Here's how the part is built. I have some questions about the finished solid (model axes, mm). Face numbers are marked on the shaded views. A direction names the side the tool comes from. Coordinates: 2 decimals unless noted, no trailing zeros. Order: outer loops, then holes, each group sorted by start corner. A loop starts at its lowest first (then second) coordinate and runs counter-clockwise, first axis right, second up. Notation, with made-up numbers: (-3, 2) - (4, 2) arc R34 ccw to (4, 33) - close; hole circle Ø5 at (-8, -10.5). An arc over 180 degrees is marked (long way). Answer in a Markdown table with one row per item. Add a question column.
Item 1: If I drill on line 1 along Z through (x, y) = (32, 17) (3 decimals); line 2 along Y through (x, z) = (2, -38.1) (3 decimals); line 3 along X through (y, z) = (35.5, 15.5) (3 decimals), over which ranges is the centre line in solid material (lowest first)? Write a range as from..to.
Item 2: I want a section at D-D (z = 38.1). Please give me the cut outline in (x, y) (3 decimals), plus the area to 3 significant figures.
Item 3: I want a section at A-A (z = -40). Please give me the cut outline in (x, y) (3 decimals).
Item 4: Thinking about a two-plate mould opening in Z: for the marked faces 1, 2 and 3, which applies, +Z half, -Z half, draft (parallel to the pull), parting line (faces both ways), or undercut?
Item 5: Will these pins go through, and if not, where does the flat tip stop? pin 1 Ø5 at (y, z) = (34.5, -36) entering from -X; pin 2 Ø8 at (x, z) = (22.5, 41.5) entering from +Y (3 decimals); pin 3 Ø12.5 at (y, z) = (53, 4) entering from +X (3 decimals).
Item 6: I want a section at B-B (x = 11). Please give me the cut outline in (y, z) (3 decimals).
Item 7: On a 3-axis mill with a long thin cutter (end or side, diameter ignored), from which of +Z, -Z, +X, -X, +Y, -Y can I reach the whole of each face in a straight line? I mean the marked faces 4, 5 and 6. Say none if no direction works.
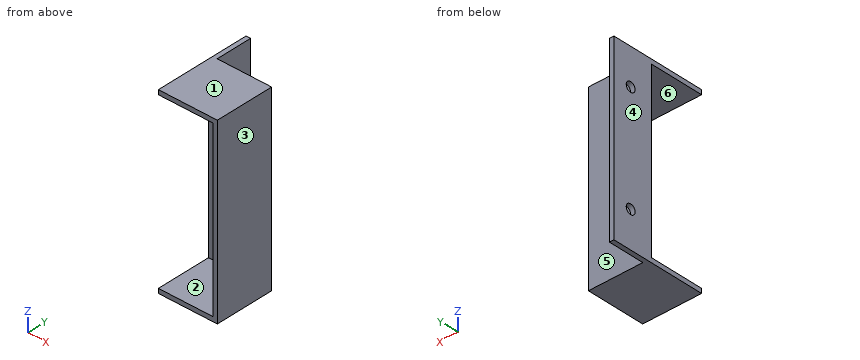
Autodesk Inventor part; units mm, degrees
ref_plane "YZ Plane" through (0, 0, 0) normal (1, 0, 0) x (0, 1, 0)
ref_plane "XZ Plane" through (0, 0, 0) normal (0, 1, 0) x (-1, 0, 0)
ref_plane "XY Plane" through (0, 0, 0) normal (0, 0, 1) x (1, 0, 0)
sketch "Sketch1" plane through (0, 0, 0) normal (0, 0, 1) x (1, 0, 0)
  line L0 (0, 66.675) -> (0, 38.1)
  line L1 (0, 66.675) -> (3.175, 66.675)
  line L2 (3.175, 66.675) -> (3.175, 41.275)
  line L3 (3.175, 41.275) -> (41.275, 41.275)
  line L4 (41.275, 41.275) -> (41.275, 0)
  line L5 (41.275, 0) -> (38.1, 0)
  line L6 (38.1, 0) -> (38.1, 38.1)
  line L7 (38.1, 38.1) -> (0, 38.1)
  point P0 (0, 0)
  dimension "d0" = 3.175
  dimension "d1" = 3.175
  dimension "d2" = 3.175
  dimension "d3" = 38.1
  dimension "d4" = 38.1
  dimension "d5" = 25.4
extrude "Extrusion1" add sketch "Sketch1" along normal mid plane 127
sketch "Sketch2" plane through (0, 0, 63.5) normal (0, 0, 1) x (1, 0, 0)
  line L0 (0, 38.1) -> (38.1, 38.1)
  line L1 (38.1, 38.1) -> (38.1, 0)
  line L2 (0, 38.1) -> (38.1, 38.1)
  line L3 (38.1, 38.1) -> (38.1, 0)
  line L4 (38.1, 0) -> (0, 0)
  line L5 (0, 0) -> (0, 38.1)
  point P0 (0, 0)
extrude "Extrusion2" add sketch "Sketch2" against normal blind 3.175
sketch "Sketch3" plane through (0, 0, -63.5) normal (0, 0, -1) x (-1, 0, 0)
  line L0 (-38.1, 38.1) -> (0, 38.1)
  line L1 (0, 0) -> (0, 38.1)
  line L2 (-38.1, 38.1) -> (0, 38.1)
  line L3 (0, 38.1) -> (0, 0)
  line L4 (0, 0) -> (-38.1, 0)
  line L5 (-38.1, 0) -> (-38.1, 38.1)
extrude "Extrusion3" add sketch "Sketch3" against normal blind 3.175
sketch "Sketch4" plane through (3.175, 41.275, 63.5) normal (1, 0, 0) x (0, 0, -1)
  line L0 (0, 0) -> (0, 25.4) construction
  line L1 (0, 12.7) -> (127, 12.7) construction
  line L2 (127, 25.4) -> (127, 0) construction
  point P0 (63.5, -41.275)
  point P1 (25.4, 12.7)
  point P2 (101.6, 12.7)
  dimension "d12" = 76.2
  dimension "d13" = 25.4
hole "Hole1" at (3.175, 53.975, 38.1) at (3.175, 53.975, -38.1) direction (-1, 0, 0) diameter 6.7564 end through all
equation "\"d0\" = materialWidth"
equation "\"d1\" = materialWidth"
equation "\"d2\" = materialWidth"
equation "\"d5\" = heightForBolts"
equation "\"d6\" = overallWidth"
equation "\"d8\" = materialWidth"
equation "\"d10\" = materialWidth"
equation "\"overallWidth\" = 127"
equation "\"extendFromWall\" = 63.5"
equation "\"heightForBolts\" = 25.4"
equation "\"materialWidth\" = 3.175"
equation "\"plugHeight\" = 38.1"
equation "\"plugDepth\" = 38.1"
equation "\"distanceBetweenBolts\" = overallWidth - 2 * distanceEdgeToBoltHoles"
equation "\"distanceEdgeToBoltHoles\" = 25.4"
properties part number "electricalCover"
Values follow:
| question | item | result |
|---|---|---|
| 1 | line 1 | z = -63.5..-60.325, 60.325..63.5 |
| 1 | line 2 | y = 38.1..50.597, 57.353..66.675 |
| 1 | line 3 | x = 38.1..41.275 |
| 2 | outline | (0, 38.1) - (38.1, 38.1) - (38.1, 0) - (41.275, 0) - (41.275, 41.275) - (3.175, 41.275) - (3.175, 50.597) - (0, 50.597) - close; (0, 57.353) - (3.175, 57.353) - (3.175, 66.675) - (0, 66.675) - close |
| 2 | area | 311 mm^2 |
| 3 | outline | (0, 38.1) - (38.1, 38.1) - (38.1, 0) - (41.275, 0) - (41.275, 41.275) - (3.175, 41.275) - (3.175, 51.182) - (0, 51.182) - close; (0, 56.768) - (3.175, 56.768) - (3.175, 66.675) - (0, 66.675) - close |
| 4 | face 1 | +Z half |
| 4 | face 2 | undercut |
| 4 | face 3 | draft |
| 5 | pin 1 | stops at x = 38.1 |
| 5 | pin 2 | stops at y = 41.275 |
| 5 | pin 3 | stops at x = 3.175 |
| 6 | outline | (0, -63.5) - (41.275, -63.5) - (41.275, 63.5) - (0, 63.5) - (0, 60.325) - (38.1, 60.325) - (38.1, -60.325) - (0, -60.325) - close |
| 7 | face 4 | +Z, -Z, -X, +Y, -Y |
| 7 | face 5 | +Z, -Z, +X, +Y |
| 7 | face 6 | -X, -Y |
